```python
from build123d import *

# Parameters (mm, degrees)
EXTRUDE_1_DEPTH     = 18
SKETCH_2_W          = 21
SKETCH_2_H          = 18
EXTRUDE_2_DEPTH     = 22
SKETCH_3_W          = 15
SKETCH_3_H          = 15
CUT_EXTRUDE_1_DEPTH = 74.280283842
SKETCH_4_W          = 15
SKETCH_4_H          = 15
CUT_EXTRUDE_2_DEPTH = 58.124863238
SKETCH_5_W          = 15
SKETCH_5_H          = 15
CUT_EXTRUDE_3_DEPTH = 63.467991804
SKETCH_6_R          = 1.65
CUT_EXTRUDE_4_DEPTH = 53.784941034
SKETCH_7_R          = 1.65
CUT_EXTRUDE_5_DEPTH = 47.338428976
SKETCH_8_R          = 1.65
CUT_EXTRUDE_6_DEPTH = 63.689712075
EXTRUDE_4_DEPTH     = 3
EXTRUDE_5_DEPTH     = 3
EXTRUDE_6_DEPTH     = 3
FILLET_1_R          = 3


with BuildPart() as part:
    # 草图1 → 凸台-拉伸1 (new body)
    with BuildSketch(Plane(origin=(0, 0, 0), x_dir=(1, 0, 0), z_dir=(0, 1, 0))):
        Polygon((10.5, 9), (26.5, 9), (26.5, -9), (-26.5, -9), (-26.5, 9), (-10.5, 9), (-10.5, 31), (10.5, 31), align=None)
    extrude(amount=EXTRUDE_1_DEPTH)

    # 草图2 → 凸台-拉伸2 (add)
    with BuildSketch(Plane(origin=(0, 18, 0), x_dir=(1, 0, 0), z_dir=(0, 1, 0))):
        Rectangle(SKETCH_2_W, SKETCH_2_H)
    extrude(amount=EXTRUDE_2_DEPTH)

    # 草图3 → 切除-拉伸1 (cut, through all)
    with BuildSketch(Plane.ZY.offset(26.5)):
        with Locations((1.5, 7.5)):
            Rectangle(SKETCH_3_W, SKETCH_3_H)
    extrude(amount=-CUT_EXTRUDE_1_DEPTH, mode=Mode.SUBTRACT)

    # 草图4 → 切除-拉伸2 (cut, through all)
    with BuildSketch(Plane(origin=(0, 40, 0), x_dir=(1, 0, 0), z_dir=(0, 1, 0))):
        with Locations((0, -1.5)):
            Rectangle(SKETCH_4_W, SKETCH_4_H)
    extrude(amount=-CUT_EXTRUDE_2_DEPTH, mode=Mode.SUBTRACT)

    # 草图5 → 切除-拉伸3 (cut, through all)
    with BuildSketch(Plane(origin=(0, 0, -31), x_dir=(-1, 0, 0), z_dir=(0, 0, -1))):
        with Locations((0, 7.5)):
            Rectangle(SKETCH_5_W, SKETCH_5_H)
    extrude(amount=-CUT_EXTRUDE_3_DEPTH, mode=Mode.SUBTRACT)

    # 草图6 → 切除-拉伸4 (cut, through all)
    with BuildSketch(Plane(origin=(0, 0, -9), x_dir=(-1, 0, 0), z_dir=(0, 0, -1))):
        with Locations((-16.5, 7.5)):
            Circle(SKETCH_6_R)
        with Locations((0, 24)):
            Circle(SKETCH_6_R)
        with Locations((16.5, 7.5)):
            Circle(SKETCH_6_R)
        with Locations((0, 34)):
            Circle(SKETCH_6_R)
    extrude(amount=-CUT_EXTRUDE_4_DEPTH, mode=Mode.SUBTRACT)

    # 草图7 → 切除-拉伸5 (cut, through all)
    with BuildSketch(Plane(origin=(0, 18, 0), x_dir=(1, 0, 0), z_dir=(0, 1, 0))):
        with Locations(Location((-21.5, -1.5, 0), (0, 0, 270))):
            Circle(SKETCH_7_R)
        with Locations(Location((0, 15, 0), (0, 0, 270))):
            Circle(SKETCH_7_R)
        with Locations(Location((0, 25, 0), (0, 0, 270))):
            Circle(SKETCH_7_R)
        with Locations(Location((21.5, -1.5, 0), (0, 0, 270))):
            Circle(SKETCH_7_R)
    extrude(amount=-CUT_EXTRUDE_5_DEPTH, mode=Mode.SUBTRACT)

    # 草图8 → 切除-拉伸6 (cut, through all)
    with BuildSketch(Plane(origin=(10.5, 0, 0), x_dir=(0, 0, -1), z_dir=(1, 0, 0))):
        with Locations((-1.5, 29)):
            Circle(SKETCH_8_R)
        with Locations((20, 7.5)):
            Circle(SKETCH_8_R)
    extrude(amount=-CUT_EXTRUDE_6_DEPTH, mode=Mode.SUBTRACT)

    # 草图9 → 凸台-拉伸4 (add)
    with BuildSketch(Plane(origin=(0, 0, -9), x_dir=(-1, 0, 0), z_dir=(0, 0, -1))):
        Polygon((-10.5, 40), (-26.5, 18), (-10.5, 18), align=None)
        Polygon((10.5, 40), (26.5, 18), (10.5, 18), align=None)
    extrude(amount=-EXTRUDE_4_DEPTH)

    # 草图10 → 凸台-拉伸5 (add)
    with BuildSketch(Plane(origin=(10.5, 0, 0), x_dir=(0, 0, -1), z_dir=(1, 0, 0))):
        Polygon((9, 40), (31, 18), (9, 18), align=None)
    extrude(amount=-EXTRUDE_5_DEPTH)

    # 草图11 → 凸台-拉伸6 (add)
    with BuildSketch(Plane.ZY.offset(10.5)):
        Polygon((-9, 40), (-31, 18), (-9, 18), align=None)
    extrude(amount=-EXTRUDE_6_DEPTH)

    # 圆角1
    # the kernel refuses this fillet: 3 mm, written as the material it adds along each edge
    with BuildSketch(Plane(origin=(-13.5, 21, -3), x_dir=(0, -1, 0), z_dir=(1, 0, 0))) as fillet_1_piece_1_section:
        Polygon((0, 0), (FILLET_1_R, 0), (FILLET_1_R, FILLET_1_R), (0, FILLET_1_R), align=None)
    fillet_1_piece_1 = extrude(amount=FILLET_1_R, mode=Mode.PRIVATE)
    fillet_1_piece_1 = fillet_1_piece_1 - Plane(origin=(-13.5, 21, -3), x_dir=(0, 0.7071067811865475, 0.7071067811865475), z_dir=(1, 0, 0)) * Sphere(FILLET_1_R, mode=Mode.PRIVATE)
    add(fillet_1_piece_1)
    with BuildSketch(Plane(origin=(13.5, 21, -3), x_dir=(0, -1, 0), z_dir=(0, 0, -1))) as fillet_1_piece_2_section:
        Polygon((0, 0), (FILLET_1_R, 0), (FILLET_1_R, FILLET_1_R), (0, FILLET_1_R), align=None)
    fillet_1_piece_2 = extrude(amount=FILLET_1_R, mode=Mode.PRIVATE)
    fillet_1_piece_2 = fillet_1_piece_2 - Plane(origin=(13.5, 21, -3), x_dir=(0.7071067811865475, 0.7071067811865475, 0), z_dir=(0, 0, -1)) * Sphere(FILLET_1_R, mode=Mode.PRIVATE)
    add(fillet_1_piece_2)
    with BuildSketch(Plane(origin=(-4.5, 21, -12), x_dir=(-1, 0, 0), z_dir=(0, 0, 1))) as fillet_1_piece_3_section:
        Polygon((0, 0), (FILLET_1_R, 0), (FILLET_1_R, FILLET_1_R), (0, FILLET_1_R), align=None)
    fillet_1_piece_3 = extrude(amount=FILLET_1_R, mode=Mode.PRIVATE)
    fillet_1_piece_3 = fillet_1_piece_3 - Plane(origin=(-4.5, 21, -12), x_dir=(0.7071067811865475, 0.7071067811865475, 0), z_dir=(0, 0, 1)) * Sphere(FILLET_1_R, mode=Mode.PRIVATE)
    add(fillet_1_piece_3)
    with BuildSketch(Plane(origin=(4.5, 21, -12), x_dir=(0, 0, 1), z_dir=(1, 0, 0))) as fillet_1_piece_4_section:
        Polygon((0, 0), (FILLET_1_R, 0), (FILLET_1_R, FILLET_1_R), (0, FILLET_1_R), align=None)
    fillet_1_piece_4 = extrude(amount=FILLET_1_R, mode=Mode.PRIVATE)
    fillet_1_piece_4 = fillet_1_piece_4 - Plane(origin=(4.5, 21, -12), x_dir=(0, 0.7071067811865475, -0.7071067811865475), z_dir=(1, 0, 0)) * Sphere(FILLET_1_R, mode=Mode.PRIVATE)
    add(fillet_1_piece_4)
    with BuildSketch(Plane(origin=(-10.5, 18, 9), x_dir=(-1, 0, 0), z_dir=(0, 0, -1))) as fillet_1_piece_5:
        with BuildLine():
            CenterArc((FILLET_1_R, FILLET_1_R), FILLET_1_R, 180, 90)
            Line((0, FILLET_1_R), (0, 0))
            Line((0, 0), (FILLET_1_R, 0))
        make_face()
    extrude(amount=12)
    with BuildSketch(Plane(origin=(10.5, 21, -6), x_dir=(0, 0, 1), z_dir=(0, 1, 0))) as fillet_1_piece_6_section:
        with BuildLine():
            CenterArc((FILLET_1_R, FILLET_1_R), FILLET_1_R, 180, 90)
            Line((0, FILLET_1_R), (0, 0))
            Line((0, 0), (FILLET_1_R, 0))
        make_face()
    fillet_1_piece_6 = extrude(amount=19, mode=Mode.PRIVATE)
    fillet_1_piece_6 = split(fillet_1_piece_6, bisect_by=Plane(origin=(15.455477793, 33.186218035, -5.302148296), z_dir=(-0.8087360843031884, -0.5881716976750465, 0)), keep=Keep.TOP, mode=Mode.PRIVATE)
    add(fillet_1_piece_6)
    with BuildSketch(Plane(origin=(26.5, 18, -6), x_dir=(0, 1, 0), z_dir=(-1, 0, 0))) as fillet_1_piece_7_section:
        with BuildLine():
            CenterArc((FILLET_1_R, -FILLET_1_R), FILLET_1_R, 90, 90)
            Line((0, -FILLET_1_R), (0, 0))
            Line((0, 0), (FILLET_1_R, 0))
        make_face()
    fillet_1_piece_7 = extrude(amount=13, mode=Mode.PRIVATE)
    fillet_1_piece_7 = split(fillet_1_piece_7, bisect_by=Plane(origin=(23.857097581, 21.633990826, -5.306552659), z_dir=(-0.8087360843031884, -0.5881716976750465, 0)), keep=Keep.TOP, mode=Mode.PRIVATE)
    add(fillet_1_piece_7)
    with BuildSketch(Plane(origin=(-10.5, 0, -9), x_dir=(0, 0, -1), z_dir=(0, 1, 0))) as fillet_1_piece_8_section:
        with BuildLine():
            CenterArc((FILLET_1_R, FILLET_1_R), FILLET_1_R, 180, 90)
            Line((0, FILLET_1_R), (0, 0))
            Line((0, 0), (FILLET_1_R, 0))
        make_face()
    fillet_1_piece_8 = extrude(amount=47.5, mode=Mode.PRIVATE)
    fillet_1_piece_8 = split(fillet_1_piece_8, bisect_by=Plane(origin=(-11.170543691, 29.3263589, -19.6736411), z_dir=(0, -0.7071067811865478, 0.7071067811865474)), keep=Keep.TOP, mode=Mode.PRIVATE)
    fillet_1_piece_8 = split(fillet_1_piece_8, bisect_by=Plane(origin=(-20.564055467, 26.161923732, -9.677561004), z_dir=(0.8087360843031883, -0.5881716976750465, 0)), keep=Keep.TOP, mode=Mode.PRIVATE)
    add(fillet_1_piece_8)
    with BuildSketch(Plane(origin=(10.5, 0, -9), x_dir=(1, 0, 0), z_dir=(0, 1, 0))) as fillet_1_piece_9_section:
        with BuildLine():
            CenterArc((FILLET_1_R, FILLET_1_R), FILLET_1_R, 180, 90)
            Line((0, FILLET_1_R), (0, 0))
            Line((0, 0), (FILLET_1_R, 0))
        make_face()
    fillet_1_piece_9 = extrude(amount=47.5, mode=Mode.PRIVATE)
    fillet_1_piece_9 = split(fillet_1_piece_9, bisect_by=Plane(origin=(20.564055468, 26.161923731, -9.677561004), z_dir=(-0.8087360843031884, -0.5881716976750465, 0)), keep=Keep.TOP, mode=Mode.PRIVATE)
    fillet_1_piece_9 = split(fillet_1_piece_9, bisect_by=Plane(origin=(11.170543691, 29.326358899, -19.673641101), z_dir=(0, -0.7071067811865478, 0.7071067811865474)), keep=Keep.TOP, mode=Mode.PRIVATE)
    add(fillet_1_piece_9)
    with BuildSketch(Plane(origin=(-10.5, 21, -6), x_dir=(-1, 0, 0), z_dir=(0, 1, 0))) as fillet_1_piece_10_section:
        with BuildLine():
            CenterArc((FILLET_1_R, FILLET_1_R), FILLET_1_R, 180, 90)
            Line((0, FILLET_1_R), (0, 0))
            Line((0, 0), (FILLET_1_R, 0))
        make_face()
    fillet_1_piece_10 = extrude(amount=19, mode=Mode.PRIVATE)
    fillet_1_piece_10 = split(fillet_1_piece_10, bisect_by=Plane(origin=(-15.455477793, 33.186218035, -5.302148296), z_dir=(0.8087360843031883, -0.5881716976750465, 0)), keep=Keep.TOP, mode=Mode.PRIVATE)
    add(fillet_1_piece_10)
    with BuildSketch(Plane(origin=(-26.5, 18, -6), x_dir=(0, 0, 1), z_dir=(1, 0, 0))) as fillet_1_piece_11_section:
        with BuildLine():
            CenterArc((FILLET_1_R, -FILLET_1_R), FILLET_1_R, 90, 90)
            Line((0, -FILLET_1_R), (0, 0))
            Line((0, 0), (FILLET_1_R, 0))
        make_face()
    fillet_1_piece_11 = extrude(amount=13, mode=Mode.PRIVATE)
    fillet_1_piece_11 = split(fillet_1_piece_11, bisect_by=Plane(origin=(-23.857097581, 21.633990826, -5.306552659), z_dir=(0.8087360843031883, -0.5881716976750465, 0)), keep=Keep.TOP, mode=Mode.PRIVATE)
    add(fillet_1_piece_11)
    with BuildSketch(Plane(origin=(-4.5, 18, -9), x_dir=(0, 0, -1), z_dir=(1, 0, 0))) as fillet_1_piece_12:
        with BuildLine():
            CenterArc((FILLET_1_R, FILLET_1_R), FILLET_1_R, 180, 90)
            Line((0, FILLET_1_R), (0, 0))
            Line((0, 0), (FILLET_1_R, 0))
        make_face()
    extrude(amount=9)
    with BuildSketch(Plane(origin=(7.5, 21, -9), x_dir=(0, 0, -1), z_dir=(0, 1, 0))) as fillet_1_piece_13_section:
        with BuildLine():
            CenterArc((FILLET_1_R, FILLET_1_R), FILLET_1_R, 180, 90)
            Line((0, FILLET_1_R), (0, 0))
            Line((0, 0), (FILLET_1_R, 0))
        make_face()
    fillet_1_piece_13 = extrude(amount=19, mode=Mode.PRIVATE)
    fillet_1_piece_13 = split(fillet_1_piece_13, bisect_by=Plane(origin=(6.80742854, 34.757043793, -14.242956207), z_dir=(0, -0.7071067811865478, 0.7071067811865474)), keep=Keep.TOP, mode=Mode.PRIVATE)
    add(fillet_1_piece_13)
    with BuildSketch(Plane(origin=(7.5, 18, -31), x_dir=(-1, 0, 0), z_dir=(0, 0, 1))) as fillet_1_piece_14_section:
        with BuildLine():
            CenterArc((FILLET_1_R, -FILLET_1_R), FILLET_1_R, 90, 90)
            Line((0, -FILLET_1_R), (0, 0))
            Line((0, 0), (FILLET_1_R, 0))
        make_face()
    fillet_1_piece_14 = extrude(amount=19, mode=Mode.PRIVATE)
    fillet_1_piece_14 = split(fillet_1_piece_14, bisect_by=Plane(origin=(6.80742854, 23.242956207, -25.757043793), z_dir=(0, -0.7071067811865478, 0.7071067811865474)), keep=Keep.TOP, mode=Mode.PRIVATE)
    add(fillet_1_piece_14)
    with BuildSketch(Plane(origin=(-7.5, 21, -9), x_dir=(1, 0, 0), z_dir=(0, 1, 0))) as fillet_1_piece_15_section:
        with BuildLine():
            CenterArc((FILLET_1_R, FILLET_1_R), FILLET_1_R, 180, 90)
            Line((0, FILLET_1_R), (0, 0))
            Line((0, 0), (FILLET_1_R, 0))
        make_face()
    fillet_1_piece_15 = extrude(amount=19, mode=Mode.PRIVATE)
    fillet_1_piece_15 = split(fillet_1_piece_15, bisect_by=Plane(origin=(-6.80742854, 34.757043793, -14.242956207), z_dir=(0, -0.7071067811865478, 0.7071067811865474)), keep=Keep.TOP, mode=Mode.PRIVATE)
    add(fillet_1_piece_15)
    with BuildSketch(Plane(origin=(-7.5, 18, -31), x_dir=(1, 0, 0), z_dir=(0, 0, 1))) as fillet_1_piece_16_section:
        with BuildLine():
            CenterArc((FILLET_1_R, FILLET_1_R), FILLET_1_R, 180, 90)
            Line((0, FILLET_1_R), (0, 0))
            Line((0, 0), (FILLET_1_R, 0))
        make_face()
    fillet_1_piece_16 = extrude(amount=19, mode=Mode.PRIVATE)
    fillet_1_piece_16 = split(fillet_1_piece_16, bisect_by=Plane(origin=(-6.80742854, 23.242956207, -25.757043793), z_dir=(0, -0.7071067811865478, 0.7071067811865474)), keep=Keep.TOP, mode=Mode.PRIVATE)
    add(fillet_1_piece_16)
    with BuildSketch(Plane(origin=(10.5, 18, -3), x_dir=(0, 1, 0), z_dir=(0, 0, 1))) as fillet_1_piece_17:
        with BuildLine():
            CenterArc((FILLET_1_R, -FILLET_1_R), FILLET_1_R, 90, 90)
            Line((0, -FILLET_1_R), (0, 0))
            Line((0, 0), (FILLET_1_R, 0))
        make_face()
    extrude(amount=12)


solid = part.part
```
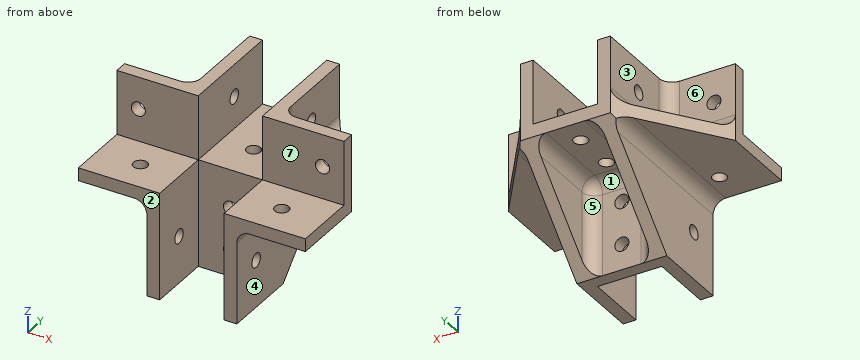
Source: CAD feature listing. Evaluate the final solid. Frame: model axes, mm. Face numbers are marked on the shaded views. A direction names the side the tool comes from. Coordinates: 2 decimals unless noted, no trailing zeros. Write each loop counter-clockwise with the first axis right and the second up, starting at its lowest first coordinate (ties: lowest second). Pieces come first, ordered by that corner, then holes. Notation, with made-up numbers: (-24, 1.5) -> (31, 1.5) arc R15 cw to (31, 7.5) -> close; hole circle Ø8 at (61, 72). An arc over 180 degrees is marked (long way). Return JSON: item names as keys, results as strings. Group by question number.
1) Section query C-C, the plane y = 7.5. State how many separate pieces and enclosed holes the cut face has, plus the area to 3 significant figures.
2) Section query A-A, the plane z = -15. Return loops of the section in (x, y), plus the area to 3 significant figures.
3) Section query D-D, the plane z = -20. Return loops of the section in (x, y).
4) Section query B-B, the plane x = -16.5. Return loops of the section in (y, z), plus the area to 3 significant figures.
5) Set-up query: the marked faces 5, 6 and 7. Return all of +Z, -Z, +X, -X, +Y, -Y with unobstructed straight access to the full face (end or side cutting, diameter ignored); none if empty.
6) Mould query, pull axis X, two halves, no side actions, for the marked faces 1, 2, 3 and 4. Classes: +X half, -X half, draft (parallel to the pull), parting line (faces both ways), or undercut.
7) Ray query, line 1 along Y through (x, z) = (0, -7); line 2 along X through (y, z) = (7, -7); line 3 along X through (y, z) = (34, -13). Return the intervals inside material, ascending.
8) Contact query for flat-ended pins moving along their axis: P1, Ø3, axis at y = 29, z = 1.5, coming from the +X side; P2, Ø10, axis at x = 5, z = -18, coming from the -Y side; P3, Ø5.5, axis at x = 16.5, y = 7.5, coming from the -Z side; P4, Ø10, axis at x = 6, z = -15, coming from the +Y side. Output: stop coordinate, or through.
From the geometry:
{
 "1": {"separate pieces": "6", "enclosed holes": "0", "area": "210 mm²"},
 "2": {"outline": "(-10.5, 0) -> (-7.5, 0) -> (-7.5, 15) -> (-1.65, 15) -> (-1.65, 18) -> (-4.5, 18) arc R3 cw to (-7.5, 21) -> (-7.5, 34) -> (-10.5, 34) -> close; (1.65, 15) -> (7.5, 15) -> (7.5, 0) -> (10.5, 0) -> (10.5, 34) -> (7.5, 34) -> (7.5, 21) arc R3 cw to (4.5, 18) -> (1.65, 18) -> close", "area": "243 mm²"},
 "3": {"outline": "(-10.5, 0) -> (-7.5, 0) -> (-7.5, 5.85) -> (-10.5, 5.85) -> close; (-10.5, 9.15) -> (-7.5, 9.15) -> (-7.5, 15) -> (7.5, 15) -> (7.5, 9.15) -> (10.5, 9.15) -> (10.5, 29) -> (7.5, 29) -> (7.5, 21) arc R3 cw to (4.5, 18) -> (-4.5, 18) arc R3 cw to (-7.5, 21) -> (-7.5, 29) -> (-10.5, 29) -> close; (7.5, 0) -> (10.5, 0) -> (10.5, 5.85) -> (7.5, 5.85) -> close"},
 "4": {"outline": "(0, -9) -> (5.85, -9) -> (5.85, -6) -> (0, -6) -> close; (9.15, -9) -> (31.75, -9) -> (31.75, -6) -> (21, -6) arc R3 cw to (18, -3) -> (18, 9) -> (15, 9) -> (15, -6) -> (9.15, -6) -> close", "area": "132 mm²"},
 "5": {"face 5": "-Z, +Y", "face 6": "+Z, -X, +Y", "face 7": "+Z, +X, -X, -Y"},
 "6": {"face 1": "undercut", "face 2": "draft", "face 3": "-X half", "face 4": "+X half"},
 "7": {"line 1": "15 to 22.35, 25.65 to 32.35, 35.65 to 40", "line 2": "-26.5 to -18.07, -14.93 to -7.5, 7.5 to 14.93, 18.07 to 26.5", "line 3": "-10.5 to -7.5, 7.5 to 10.5"},
 "8": {"P1": "through", "P2": "y = 0", "P3": "z = -9", "P4": "y = 38.94"}
}
